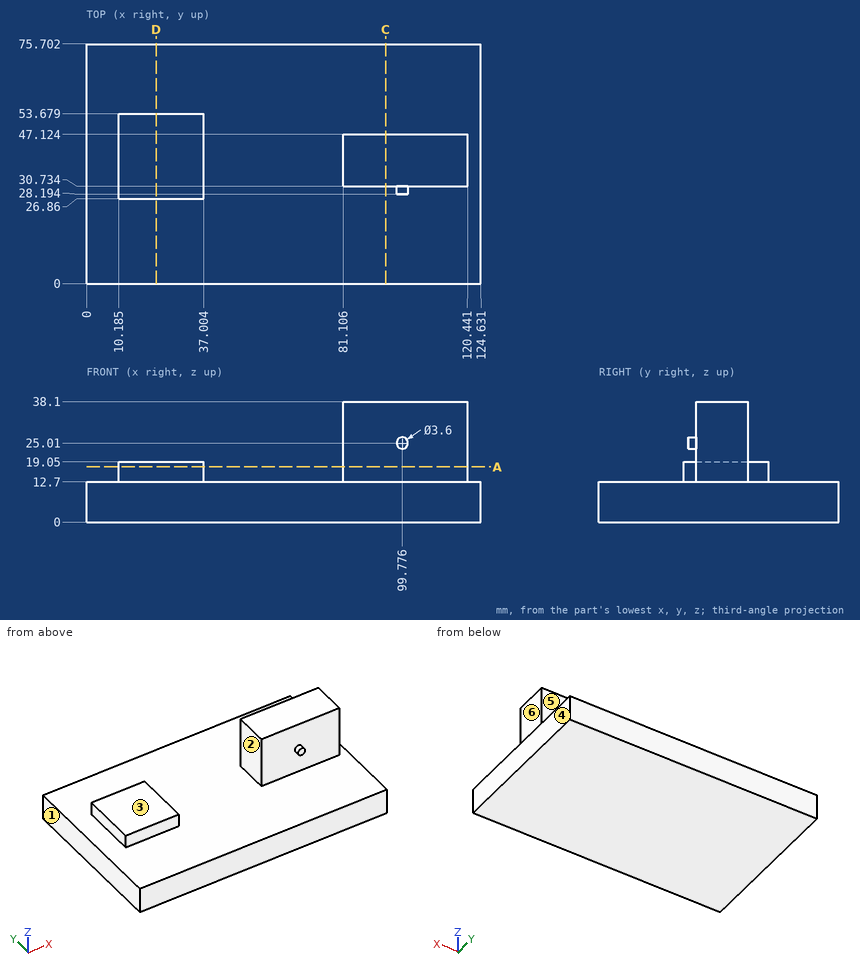
Verification items for this drawing (mm, ordinates from the low corner). A direction names the side the tool comes from. Round coordinates to 2 decimals unless told otherwise and drop trailing zeros. Write each loop counter-clockwise with the first axis right and the second up, starting at its lowest first coordinate (ties: lowest second). Pieces come first, ordered by that corner, then holes. Notation, with made-up numbers: (15, 80) - (59, 80) arc R8 ccw to (59, 85) - close; hole circle Ø11 at (23, -35). An arc over 180 degrees is marked (long way). Answer as a JSON object with one key per item and string values. Group by question number.
Q1. Section check C-C, the plane x = 94.5. Enter the section's corners in (y, z) (1 decimal).
Q2. Section check A-A, the plane z = 17.5. Enter the section's corners in (x, y) (1 decimal), plus the area to 3 significant figures.
Q3. Thickness scan on line 1 (X direction, y = 46, z = 18.5) (1 decimal); line 2 (Y direction, x = 90, z = 15.5) (1 decimal); line 3 (Z direction, x = 31, y = 18). Record the ranges inside material, lowest first.
Q4. Mould release check, pull along X, two halves, no side actions. Record for the marked faces 1, 2 and 3: released by +X, released by -X, zero draft, split by the parting line, or undercut.
Q5. Section check D-D, the plane x = 22. Enter the section's corners in (y, z), plus the area to 3 significant figures.
Q6. Go/stop test with flat-tipped pins: pin 1 Ø8 at (x, y) = (60.5, 28.5) entering from +Z; pin 2 Ø7.5 at (x, z) = (97.5, 29) entering from +Y; pin 3 Ø3 at (y, z) = (46, 14.5) entering from +X. Record where each tip stops, or that it passes through.
Q7. Tool access check on the marked faces 4, 5 and 6. Record the directions out of +Z, -Z, +X, -X, +Y, -Y that give a thin tool (end or side, any length) a straight path to the whole face; none if there is none.
Found:
{
 "1": {"outline": "(0, 0) - (75.7, 0) - (75.7, 12.7) - (47.1, 12.7) - (47.1, 38.1) - (30.7, 38.1) - (30.7, 12.7) - (0, 12.7) - close"},
 "2": {"outline": "(10.2, 26.9) - (37, 26.9) - (37, 53.7) - (10.2, 53.7) - close; (81.1, 30.7) - (120.4, 30.7) - (120.4, 47.1) - (81.1, 47.1) - close", "area": "1,360 mm^2"},
 "3": {"line 1": "x = 10.2 to 37, 81.1 to 120.4", "line 2": "y = 30.7 to 47.1", "line 3": "z = 0 to 12.7"},
 "4": {"face 1": "released by -X", "face 2": "undercut", "face 3": "zero draft"},
 "5": {"outline": "(0, 0) - (75.7, 0) - (75.7, 12.7) - (53.68, 12.7) - (53.68, 19.05) - (26.86, 19.05) - (26.86, 12.7) - (0, 12.7) - close", "area": "1,130 mm^2"},
 "6": {"pin 1": "stops at z = 12.7", "pin 2": "stops at y = 47.12", "pin 3": "stops at x = 120.44"},
 "7": {"face 4": "+Z, -Z, +X, +Y, -Y", "face 5": "+Z, +X, +Y", "face 6": "+Z, +X, +Y, -Y"}
}
